Can you work these out from the model? Positions are in its coordinate system, mm. Face numbers are marked on the shaded views. A direction names the side the tool comes from. Coordinates: 2 decimals unless noted, no trailing zeros. Loops run counter-clockwise (first coordinate to the right, second up) from the corner with the lowest first, then second, coordinate; pieces in that order, holes last.
```python
from build123d import *

# Parameters (mm, degrees)
SKETCH2_W           = 22.7
SKETCH2_H           = 22
BOSS_EXTRUDE1_DEPTH = 19
SKETCH3_R           = 0.5
BOSS_EXTRUDE2_DEPTH = 5
SKETCH5_W           = 22.7
SKETCH5_H           = 19
SKETCH5_W_2         = 16.7
SKETCH5_H_2         = 12.996403956
CUT_EXTRUDE1_DEPTH  = 5


with BuildPart() as part:
    # Sketch2 → Boss-Extrude1 (new body)
    with BuildSketch(Plane.XY):
        with Locations((11.35, -11)):
            Rectangle(SKETCH2_W, SKETCH2_H)
    extrude(amount=BOSS_EXTRUDE1_DEPTH)

    # Sketch3 → Boss-Extrude2 (add)
    with BuildSketch(Plane.XZ.offset(22)):
        with Locations(Location((18.85, 17, 0), (0, 0, 90))):
            Circle(SKETCH3_R)
        with Locations(Location((3.85, 17, 0), (0, 0, 90))):
            Circle(SKETCH3_R)
        with Locations(Location((8.85, 2, 0), (0, 0, 90))):
            Circle(SKETCH3_R)
        with Locations(Location((13.85, 2, 0), (0, 0, 90))):
            Circle(SKETCH3_R)
    extrude(amount=BOSS_EXTRUDE2_DEPTH)

    # Sketch5 → Cut-Extrude1 (cut)
    with BuildSketch(Plane(origin=(0, 0, 0), x_dir=(1, 0, 0), z_dir=(0, 1, 0))):
        with Locations((11.35, -9.5)):
            Rectangle(SKETCH5_W, SKETCH5_H)
        with Locations((11.35, -9.501798022)):
            Rectangle(SKETCH5_W_2, SKETCH5_H_2, mode=Mode.SUBTRACT)
    extrude(amount=-CUT_EXTRUDE1_DEPTH, mode=Mode.SUBTRACT)


solid = part.part
```
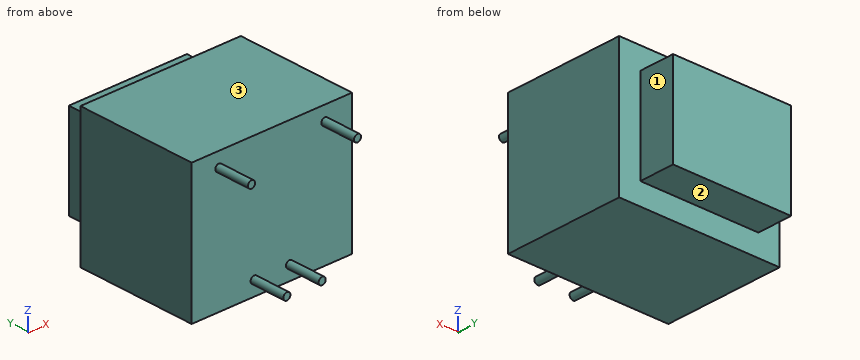
(1) I'm going to push flat-ended pins straight in: pin 1 (5.5 mm diameter, centred on x = 8.5, y = -2, fed in from +Z); pin 2 (1.5 mm diameter, centred on x = 9.5, y = -3, fed in from -Z); pin 3 (1.5 mm diameter, centred on x = 4, z = 11, fed in from -Y). Where does each tip first touch, or does it pass through?
Check values:
pin 1: stops at z = 16
pin 2: stops at z = 3
pin 3: stops at y = -22
(2) Which directions (+Z, -Z, +X, -X, +Y, -Y) give clear straight access to the entire face, cutting with the end or side of a thin tool? Please do the marked faces 1, 2 and 3.
Check values:
face 1: +Z, -Z, +X, +Y
face 2: -Z, +X, -X, +Y
face 3: +Z, +X, -X, +Y, -Y
(3) I want a section at D-D on z = 7. Write out the boundary of the cut face in (x, y), then the cut area to 3 significant figures.
Check values:
outline: (0, -22) - (22.7, -22) - (22.7, -5) - (19.7, -5) - (19.7, 0) - (3, 0) - (3, -5) - (0, -5) - close
area: 469 mm2
(4) I want a section at B-B on z = 2. Write out the boundary of the cut face in (x, y).
Check values:
outline: (0, -22) - (8.35, -22) - (8.35, -27) - (9.35, -27) - (9.35, -22) - (13.35, -22) - (13.35, -27) - (14.35, -27) - (14.35, -22) - (22.7, -22) - (22.7, -5) - (0, -5) - close
(5) I want a section at C-C on y = -22.5. Write out the boundary of the cut face in (x, z), then the cut area to 3 significant figures.
Check values:
outline: circle Ø1 at (3.85, 17); circle Ø1 at (8.85, 2); circle Ø1 at (13.85, 2); circle Ø1 at (18.85, 17)
area: 3.14 mm2
(6) If I drill on probe 1 along Y at (x, z) = (7.5, 7.5); probe 2 along Z at (x, y) = (17.5, -2.5); probe 3 along Y at (x, z) = (11.75, 2.75), over which ranges is the centre line in solid material (lowest first)?
Check values:
probe 1: y = -22 to 0
probe 2: z = 3 to 16
probe 3: y = -22 to -5
(7) I want a section at A-A on x = 18.85. Write out the boundary of the cut face in (y, z).
Check values:
outline: (-27, 16.5) - (-22, 16.5) - (-22, 0) - (-5, 0) - (-5, 3) - (0, 3) - (0, 16) - (-5, 16) - (-5, 19) - (-22, 19) - (-22, 17.5) - (-27, 17.5) - close
